Autodesk Inventor part; units mm, degrees
ref_plane "MidSidePlane" through (0, 0, 10) normal (0, 0, 1) x (1, 0, 0)
ref_plane "YZ Plane" through (0, 0, 0) normal (1, 0, 0) x (0, 1, 0)
ref_plane "XZ Plane" through (0, 0, 0) normal (0, 1, 0) x (-1, 0, 0)
sketch "ShaftProfile" plane through (0, 0, 0) normal (0, 0, 1) x (1, 0, 0)
  line L0 (-48, 0) -> (22, 0) construction
  line L1 (-38, 9) -> (12, 9)
  line L2 (12, 9) -> (12, 0)
  line L3 (-38, 0) -> (-38, 9)
  line L4 (-38, 0) -> (12, 0)
  point P0 (0, 0)
  dimension "d1" = 50
  dimension "d2" = 9
  dimension "d4" = 38
revolve "ShaftFeature" add sketch "ShaftProfile" angle 360 about axis through (-38, 0, 0) along (1, 0, 0)
sketch "Sketch2" plane through (-38, 0, 0) normal (-1, 0, 0) x (0, 0, 1)
  circle A0 centre (0, 0) radius 9
hole "ShaftHoleFeature" at (-38, 0, 0) direction (1, 0, 0) diameter 16 end through all
ref_plane "MidSidePlane" through (0, 0, 10) normal (0, 0, 1) x (1, 0, 0)
sketch "CapHoles" plane through (0, 0, 10) normal (0, 0, 1) x (1, 0, 0)
  line L0 (12, -9) -> (12, 9) construction
  line L1 (-38, -9) -> (-38, 9) construction
  line L2 (-58, 0) -> (82, 0) construction
  circle A0 centre (-33.5, 0) radius 1.25
  circle A1 centre (7.5, 0) radius 1.25
  dimension "d24" = 2.5
  dimension "d25" = 4.5
  dimension "d26" = 4.5
extrude "CapHolesFeature" cut sketch "CapHoles" against normal through all
equation "\"d26\" = d25"
properties part number "BackPair1PistonShaft"
Build history of the part. All positions in model axes, mm. Coordinates: 2 decimals unless noted, no trailing zeros. Order: outer loops, then holes, each group sorted by start corner. A loop starts at its lowest first (then second) coordinate and runs counter-clockwise, first axis right, second up. Notation, with made-up numbers: (-2, -14.5) -> (17, -14.5) arc R24 ccw to (17, 6.5) -> close; hole circle Ø5 at (6, -19.75). An arc over 180 degrees is marked (long way). Answer in a Markdown table with one row per item. Add a question column.
Q1. Band-saw the part on D-D, the plane x = -4. List the corners of the cut face in (y, z), then the cut area to 3 significant figures.
Q2. Wall check: line 1 along X through (y, z) = (0, 8.2); line 2 along Z through (x, y) = (-19, 0); line 3 along Z through (x, y) = (1.5, -3.25). Give the ranges that are in metal, low to high. Write a range as [from, to].
Q3. Band-saw the part on A-A, the plane y = 0. List the corners of the cut face in (x, z).
Q4. Mould opens along Y. For faces 1 (the face through (8.172, 1.054, -8.443)), 2 (the face through (-12.65, -1.172, 8.923)) say: +Y half, -Y half, draft (parallel to the pull), parting line (faces both ways), or undercut.
Q5. Band-saw the part on B-B, the plane z = 0. List the corners of the cut face in (x, y), then the cut area to 3 significant figures.
Q6. Drop flat-ended pins along their axis: pin 1 (1.5 mm diameter, centred on x = -29.5, y = 5, fed in from +Z); pin 2 (4 mm diameter, centred on x = -1.5, z = 4.5, fed in from -Y); pin 3 (5 mm diameter, centred on x = -22, y = 5, fed in from -Z). Give the stop position or say it passes through.
Q7. Band-saw the part on C-C, the plane x = 7.5. List the corners of the cut face in (y, z), then the cut area to 3 significant figures.
Answers follow:
| question | item | result |
|---|---|---|
| 1 | outline | circle Ø18 at (0, 0); hole circle Ø16 at (0, 0) |
| 1 | area | 53.4 mm^2 |
| 2 | line 1 | [-38, -34.75], [-32.25, 6.25], [8.75, 12] |
| 2 | line 2 | [-9, -8], [8, 9] |
| 2 | line 3 | [-8.39, -7.31], [7.31, 8.39] |
| 3 | outline | (-38, -9) -> (-34.75, -9) -> (-34.75, -8) -> (-38, -8) -> close; (-38, 8) -> (-34.75, 8) -> (-34.75, 9) -> (-38, 9) -> close; (-32.25, -9) -> (6.25, -9) -> (6.25, -8) -> (-32.25, -8) -> close; (-32.25, 8) -> (6.25, 8) -> (6.25, 9) -> (-32.25, 9) -> close; (8.75, -9) -> (12, -9) -> (12, -8) -> (8.75, -8) -> close; (8.75, 8) -> (12, 8) -> (12, 9) -> (8.75, 9) -> close |
| 4 | face 1 | undercut |
| 4 | face 2 | parting line |
| 5 | outline | (-38, -9) -> (12, -9) -> (12, -8) -> (-38, -8) -> close; (-38, 8) -> (12, 8) -> (12, 9) -> (-38, 9) -> close |
| 5 | area | 100 mm^2 |
| 6 | pin 1 | z = 7.93 |
| 6 | pin 2 | y = -8.65 |
| 6 | pin 3 | z = -8.65 |
| 7 | outline | (-1.25, -8.91) -> (-1.25, -7.9) arc R8 cw to (-1.25, 7.9) -> (-1.25, 8.91) arc R9 ccw to start; (1.25, -8.91) arc R9 ccw to (1.25, 8.91) -> (1.25, 7.9) arc R8 cw to (1.25, -7.9) -> close |
| 7 | area | 48.4 mm^2 |
